```python
from build123d import *

# Parameters (mm, degrees)
SKETCH3_W               = 5
SKETCH3_H               = 2.15
SKETCH4_W               = 5
SKETCH4_H               = 2.15
CUT_EXTRUDE1_DEPTH      = 7.5
CUT_EXTRUDE1_DEPTH_BACK = 7.5
SKETCH5_W               = 30
SKETCH5_H               = 90
SKETCH5_W_2             = 15
SKETCH5_H_2             = 60


with BuildPart() as part:
    # Sketch1 → Revolve1 (revolve)
    with BuildSketch(Plane.XY, mode=Mode.PRIVATE) as revolve1_sk:
        with BuildLine():
            Line((0, 0), (0, 14.5))
            Line((0, 14.5), (0.5, 15))
            Line((0.5, 15), (4.5, 15))
            Line((4.5, 15), (5, 14.5))
            Line((5, 14.5), (5, 7.9))
            ThreePointArc((5, 7.9), (5.117157288, 7.617157288), (5.4, 7.5))
            Line((5.4, 7.5), (19.5, 7.5))
            Line((19.5, 7.5), (20, 7))
            Line((20, 7), (20, 0))
            Line((20, 0), (0, 0))
        make_face()
    revolve(revolve1_sk.sketch.rotate(Axis((20, 0, 0), (-1, 0, 0)), 270), axis=Axis((20, 0, 0), (-1, 0, 0)))

    # Sketch2 → Cut-Revolve1 (revolve, cut)
    with BuildSketch(Plane.XY, mode=Mode.PRIVATE) as cut_revolve1_sk:
        Polygon((0, 0), (0, 4), (0.75, 3.25), (19.25, 3.25), (20, 4), (20, 0), align=None)
    revolve(cut_revolve1_sk.sketch.rotate(Axis((20, 0, 0), (-1, 0, 0)), 270), axis=Axis((20, 0, 0), (-1, 0, 0)), mode=Mode.SUBTRACT)

    # Sketch3 → Cut-Revolve2 (revolve, cut)
    with BuildSketch(Plane.XY, mode=Mode.PRIVATE) as cut_revolve2_sk:
        with Locations((2.5, 12.075)):
            Rectangle(SKETCH3_W, SKETCH3_H)
    revolve(cut_revolve2_sk.sketch.rotate(Axis((5, 11, 0), (-1, 0, 0)), 270), axis=Axis((5, 11, 0), (-1, 0, 0)), mode=Mode.SUBTRACT)

    # Sketch4 → Cut-Revolve3 (revolve, cut)
    with BuildSketch(Plane.XY, mode=Mode.PRIVATE) as cut_revolve3_sk:
        with Locations((2.5, -9.925)):
            Rectangle(SKETCH4_W, SKETCH4_H)
    revolve(cut_revolve3_sk.sketch.rotate(Axis((5, -11, 0), (-1, 0, 0)), 270), axis=Axis((5, -11, 0), (-1, 0, 0)), mode=Mode.SUBTRACT)

    # Sketch5 → Cut-Extrude1 (cut, two sides: drawn at the far end of the back side and taken through both)
    with BuildSketch(Plane(origin=(0, 0, 0), x_dir=(0, 0, -1), z_dir=(1, 0, 0)).offset(-CUT_EXTRUDE1_DEPTH_BACK)):
        Rectangle(SKETCH5_W, SKETCH5_H)
        Rectangle(SKETCH5_W_2, SKETCH5_H_2, mode=Mode.SUBTRACT)
    extrude(amount=CUT_EXTRUDE1_DEPTH + CUT_EXTRUDE1_DEPTH_BACK, mode=Mode.SUBTRACT)


solid = part.part
```
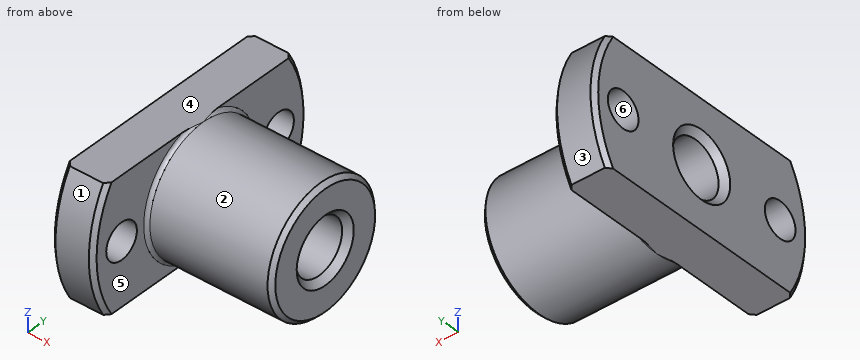
Geometry check sheet. Reference: the model listing, model coordinates, mm. Face numbers are marked on the shaded views. A direction names the side the tool comes from. Round coordinates to 2 decimals unless told otherwise and drop trailing zeros. Order: outer loops, then holes, each group sorted by start corner. A loop starts at its lowest first (then second) coordinate and runs counter-clockwise, first axis right, second up. Notation, with made-up numbers: M -39.75,77.25 L -34.75,77.25 A16 ccw -34.75,89.25 Z; hole C -39.75,40 d8. An arc over 180 degrees is marked long. Answer as CSV lines item,"result".
1) Sectioned sample at B-B on y = -11. Record the cut outline in (x, z).
Entries:
outline,"M 0,-7.5 L 5,-7.5 L 5,-2.15 L 0,-2.15 Z; M 0,2.15 L 5,2.15 L 5,7.5 L 0,7.5 Z"
2) Sectioned sample at C-C on x = 4. Record the cut outline in (y, z).
Entries:
outline,"M -12.99,-7.5 L 12.99,-7.5 A15 ccw 12.99,7.5 L -12.99,7.5 A15 ccw Z; hole C -11,0 d4.3; hole C 0,0 d6.5; hole C 11,0 d4.3"
3) Sectioned sample at A-A on z = 0. Give the number of separate pieces and of enclosed holes in the cut face, and give its area (3 significant figures).
Entries:
separate pieces,"4"
enclosed holes,"0"
area,"200 mm2"
4) Gauge pin test, flat ends, axial feed: pin 1 Ø4 at (y, z) = (5, 5.5) entering from +X; pin 2 Ø3.5 at (y, z) = (10, 1) entering from +X; pin 3 Ø8 at (x, z) = (10.5, -1.5) entering from -Y; pin 4 Ø8 at (x, z) = (7.5, 5.5) entering from +Y. Record the tip position at first contact, or that the pin passes through.
Entries:
pin 1,"x = 20"
pin 2,"x = 5"
pin 3,"y = -7.5"
pin 4,"y = 14.73"
5) Sectioned sample at D-D on x = 11.5. Record the cut outline in (y, z), and give its area (3 significant figures).
Entries:
outline,"C 0,0 d15; hole C 0,0 d6.5"
area,"144 mm2"
6) Thickness scan on probe 1 along Y at (x, z) = (2.45, 0); probe 2 along X at (y, z) = (13.5, 1.75); probe 3 along Y at (x, z) = (15, 0). Record the ranges inside material, lowest first. Write a range as [from, to].
Entries:
probe 1,"[-15, -13.15], [-8.85, -3.25], [3.25, 8.85], [13.15, 15]"
probe 2,"[0, 5]"
probe 3,"[-7.5, -3.25], [3.25, 7.5]"
7) Tool access check on the marked faces 1 and 2. Record the directions out of +Z, -Z, +X, -X, +Y, -Y that give a thin tool (end or side, any length) a straight path to the whole face; none if there is none.
Entries:
face 1,"+X, -X, -Y"
face 2,"+X"
8) Mould release check, pull along Z, two halves, no side actions. Record for the marked faces 3, 4, 5 and 6: +Z half, -Z half, draft (parallel to the pull), parting line (faces both ways), or undercut.
Entries:
face 3,"parting line"
face 4,"+Z half"
face 5,"draft"
face 6,"undercut"
